Design review of the part built by this model. Coordinates are the model's own, in mm. A direction names the side the tool comes from. Coordinates: 2 decimals unless noted, no trailing zeros. Write each loop counter-clockwise with the first axis right and the second up, starting at its lowest first coordinate (ties: lowest second). Pieces come first, ordered by that corner, then holes. Notation, with made-up numbers: M 66,87.5 L 98,87.5 A23 cw 98,126.5 Z; hole C 69.5,-31 d10. An arc over 180 degrees is marked long. Return JSON: item names as keys, results as strings. Group by question number.
```python
from build123d import *

# Parameters (mm, degrees)
EXTRUDE_1_DEPTH      = 2
HOLE_WIZARD_M2_5_1_D = 2.55
SKETCH_5_OUTSIDE_W   = 241.652
SKETCH_5_OUTSIDE_H   = 141.652
CUT_EXTRUDE_1_DEPTH  = 10
FILLET_1_R           = 3


with BuildPart() as part:
    # 草图1 → 凸台-拉伸1 (new body)
    with BuildSketch(Plane.XY):
        with BuildLine():
            Line((-50, 48), (50, 48))
            ThreePointArc((50, 48), (98, 0), (50, -48))
            Line((50, -48), (-50, -48))
            ThreePointArc((-50, -48), (-98, 0), (-50, 48))
        make_face()
    extrude(amount=EXTRUDE_1_DEPTH)

    # M2.5 螺旋的螺纹孔钻头1 (through all)
    with Locations(Plane(origin=(-89.264880132, 16.264045876, 2), x_dir=(1, 0, 0), z_dir=(0, 0, 1))):
        with Locations((0, 0), (23.000834256, 23.000834256), (55.528926008, 23.000834256), (55.528926008, -55.528926008), (23.000834256, -55.528926008), (0, -32.528091752), (79.433936211, -2.382513767), (78.529760264, -32.528091752), (100, -32.528091752), (99.095824053, -2.382513767), (178.529760264, -32.528091752), (155.528926008, -55.528926008), (123.000834256, -55.528926008), (123.000834256, 23.000834256), (155.528926008, 23.000834256), (178.529760264, 0)):
            Hole(HOLE_WIZARD_M2_5_1_D / 2)

    # 草图5 outside → 切除-拉伸1 (cut)
    with BuildSketch(Plane.XY):
        Rectangle(SKETCH_5_OUTSIDE_W, SKETCH_5_OUTSIDE_H)
        with BuildLine():
            Line((-17.624645737, -13.410310822), (-17.624645737, 13.410310822))
            ThreePointArc((-17.624645737, 13.410310822), (-19.866504602, 17.8877739), (-22.723636606, 22))
            Line((-22.723636606, 22), (-50, 22))
            Line((-50, 22), (-79.748949561, 22))
            ThreePointArc((-79.748949561, 22), (-82.205746178, 18.215101238), (-84.183542703, 14.159286998))
            ThreePointArc((-84.183542703, 14.159286998), (-91.36963901, 11.182708447), (-94.346217561, 18.368804754))
            ThreePointArc((-94.346217561, 18.368804754), (-90.27157125, 26.118969143), (-84.856850116, 33))
            Line((-84.856850116, 33), (-50, 33))
            Line((-50, 33), (-15.143149884, 33))
            ThreePointArc((-15.143149884, 33), (-9.72842875, 26.118969143), (-5.653782439, 18.368804754))
            Line((-5.653782439, 18.368804754), (5.653782439, 18.368804754))
            ThreePointArc((5.653782439, 18.368804754), (9.72842875, 26.118969143), (15.143149884, 33))
            Line((15.143149884, 33), (50, 33))
            Line((50, 33), (84.856850116, 33))
            ThreePointArc((84.856850116, 33), (90.27157125, 26.118969143), (94.346217561, 18.368804754))
            ThreePointArc((94.346217561, 18.368804754), (91.36963901, 11.182708447), (84.183542703, 14.159286998))
            ThreePointArc((84.183542703, 14.159286998), (82.205746178, 18.215101238), (79.748949561, 22))
            Line((79.748949561, 22), (50, 22))
            Line((50, 22), (22.723636606, 22))
            ThreePointArc((22.723636606, 22), (19.866504602, 17.8877739), (17.624645737, 13.410310822))
            Line((17.624645737, 13.410310822), (17.624645737, -13.410310822))
            ThreePointArc((17.624645737, -13.410310822), (19.866504602, -17.8877739), (22.723636606, -22))
            Line((22.723636606, -22), (50, -22))
            Line((50, -22), (79.748949561, -22))
            ThreePointArc((79.748949561, -22), (82.205746178, -18.215101238), (84.183542703, -14.159286998))
            ThreePointArc((84.183542703, -14.159286998), (91.36963901, -11.182708447), (94.346217561, -18.368804754))
            ThreePointArc((94.346217561, -18.368804754), (90.27157125, -26.118969143), (84.856850116, -33))
            Line((84.856850116, -33), (50, -33))
            Line((50, -33), (15.143149884, -33))
            ThreePointArc((15.143149884, -33), (9.72842875, -26.118969143), (5.653782439, -18.368804754))
            Line((5.653782439, -18.368804754), (-5.653782439, -18.368804754))
            ThreePointArc((-5.653782439, -18.368804754), (-9.72842875, -26.118969143), (-15.143149884, -33))
            Line((-15.143149884, -33), (-50, -33))
            Line((-50, -33), (-84.856850116, -33))
            ThreePointArc((-84.856850116, -33), (-90.27157125, -26.118969143), (-94.346217561, -18.368804754))
            ThreePointArc((-94.346217561, -18.368804754), (-91.36963901, -11.182708447), (-84.183542703, -14.159286998))
            ThreePointArc((-84.183542703, -14.159286998), (-82.205746178, -18.215101238), (-79.748949561, -22))
            Line((-79.748949561, -22), (-50, -22))
            Line((-50, -22), (-22.723636606, -22))
            ThreePointArc((-22.723636606, -22), (-19.866504602, -17.8877739), (-17.624645737, -13.410310822))
        make_face(mode=Mode.SUBTRACT)
    extrude(amount=CUT_EXTRUDE_1_DEPTH, mode=Mode.SUBTRACT)

    # 圆角1
    fillet_1_edges = [part.edges().sort_by_distance(p)[0] for p in [
        (5.653782439, 18.368804754, 1),
        (-5.653782439, 18.368804754, 1),
        (-15.143149884, 33, 1),
        (-84.856850116, 33, 1),
        (-79.748949561, 22, 1),
        (-22.723636606, 22, 1),
        (-17.624645737, 13.410310822, 1),
        (-17.624645737, -13.410310822, 1),
        (-22.723636606, -22, 1),
        (-79.748949561, -22, 1),
        (-84.856850116, -33, 1),
        (-15.143149884, -33, 1),
        (-5.653782439, -18.368804754, 1),
        (5.653782439, -18.368804754, 1),
        (15.143149884, -33, 1),
        (84.856850116, -33, 1),
        (79.748949561, -22, 1),
        (22.723636606, -22, 1),
        (17.624645737, -13.410310822, 1),
        (17.624645737, 13.410310822, 1),
        (22.723636606, 22, 1),
        (79.748949561, 22, 1),
        (84.856850116, 33, 1),
        (15.143149884, 33, 1),
    ]]
    fillet(fillet_1_edges, radius=FILLET_1_R)


solid = part.part
```
Item 1: Add section B-B (y = 5). Write out the cut boundary in (x, z).
Item 2: The part is to be moulded in two halves that separate along Y. For faces 1 (the cylindrical face through (-9.93, 26.43, 0.99)), 2 (the cylindrical face through (-82.6, -17.5, 1)), 3 (the cylindrical face through (9.93, -26.43, 0.99)), say which applies: pulls with the +Y half, pulls with the -Y half, needs draft (parallel to the pull), parting line crosses it, or undercut.
Item 3: For pin 1 (1 mm diameter, centred on x = 1, z = 1.5, fed in from -Y); pin 2 (0.6 mm diameter, centred on x = 0, z = 1, fed in from +Y); pin 3 (1 mm diameter, centred on y = -5, z = 1, fed in from -X), all flat-tipped, find the tip position at first contact; note any pin that passes through.
Item 4: For line 1 (Y direction, x = 75.5, z = 0.9); line 2 (X direction, y = 17, z = 1.85); line 3 (Y direction, x = 23, z = 1.85), list the stretches that pass through material, from the lowest coordinate up.
Item 5: Add section C-C (z = 1.25). Count the separate pieces of the cut face and the enclosed holes in it, plus the area to 3 significant figures.
Item 6: Machinability: for faces 4 (the cylindrical face through (19.67, 17.55, 0.99)), 5 (the cylindrical face through (-9.82, -26.26, 0.99)), 6 (the cylindrical face through (90.697, -25.45, 0.986)), which of the approach directions +Z, -Z, +X, -X, +Y, -Y give a long, thin tool a straight path to every point of the face, cutting with its end or side? Answer none if there is none.
Item 7: Add section A-A (x = 61). Write out the cut boundary in (y, z).
Geometry check:
{
 "1": {"outline": "M -17.62,0 L 17.62,0 L 17.62,2 L -17.62,2 Z"},
 "2": {"face 1": "pulls with the +Y half", "face 2": "undercut", "face 3": "pulls with the -Y half"},
 "3": {"pin 1": "y = -18.37", "pin 2": "y = 18.37", "pin 3": "x = -17.62"},
 "4": {"line 1": "-33 to -22, 22 to 33", "line 2": "-94.72 to -90.31, -88.22 to -82.86, -19.36 to 19.36, 82.86 to 88.22, 90.31 to 94.72", "line 3": "-33 to -21.75, 21.75 to 33"},
 "5": {"separate pieces": "1", "enclosed holes": "8", "area": "5,420 mm^2"},
 "6": {"face 4": "+Z, -Z", "face 5": "+Z, -Z, -Y", "face 6": "+Z, -Z, +X, -Y"},
 "7": {"outline": "M -33,0 L -22,0 L -22,2 L -33,2 Z; M 22,0 L 33,0 L 33,2 L 22,2 Z"}
}
